Verification items for the finished model (mm, model axes). A direction names the side the tool comes from. Coordinates: 2 decimals unless noted, no trailing zeros. Loops run counter-clockwise (first coordinate to the right, second up) from the corner with the lowest first, then second, coordinate; pieces in that order, holes last. Notation, with made-up numbers: (10.5, 83.5) - (32.5, 83.5) arc R22 ccw to (32.5, 110.5) - close; hole circle Ø3 at (36, 48). An arc over 180 degrees is marked (long way). Answer as CSV lines item,"result". Start each with the question number.
1. Material ranges on line 1 (Z direction, x = 12.7, y = 1.75); line 2 (Y direction, x = 7.5, z = 548) (3 decimals); line 3 (X direction, y = 23.8, z = 698.5), recorded low to high. Write a range as [from, to].
2. Release check for a two-part mould opening along X. For faces 3 (the flat face through (13, 3.175, 361)), 4 (the flat face through (24, 13, 711.2)), 5 (the flat face through (25.4, 13, 351)) record: pulls with the +X half, pulls with the -X half, needs draft (parallel to the pull), parting line crosses it, or undercut.
3. Gauge pin test, flat end, axial feed: P1, Ø4, axis at x = 12.7, z = 476.25, coming from the -Y side. Record the tip position at first contact, or that the pin passes through.
4. Cross-section at A-A (z = 141.5). Enter the section's corners in (x, y) (3 decimals).
5. Cross-section at B-B (y = 8.75). Enter the section's corners in (x, z) (3 decimals).
6. Set-up check for faces 1 (the flat face through (0, 13, 351)), 2 (the flat face through (22.225, 13, 361)): record each of +Z, -Z, +X, -X, +Y, -Y from which the full face is reachable in a straight line by a thin tool's end or side.
Autodesk Inventor part; units mm, degrees
ref_plane "YZ Plane" through (0, 0, 0) normal (1, 0, 0) x (0, 1, 0)
ref_plane "XZ Plane" through (0, 0, 0) normal (0, 1, 0) x (-1, 0, 0)
ref_plane "XY Plane" through (0, 0, 0) normal (0, 0, 1) x (1, 0, 0)
sketch "Sketch1" plane through (0, 0, 0) normal (0, 0, 1) x (1, 0, 0)
  line L0 (0, 0) -> (25.4, 0)
  line L1 (25.4, 0) -> (25.4, 25.4)
  line L2 (25.4, 25.4) -> (0, 25.4)
  line L3 (0, 25.4) -> (0, 0)
  dimension "d0" = 25.4
  dimension "d1" = 25.4
extrude "Extrusion1" add sketch "Sketch1" along normal blind 711.2
sketch "Sketch2" plane through (0, 25.4, 0) normal (0, 1, 0) x (1, 0, 0)
  line L0 (0, -711.2) -> (25.4, -711.2) construction
  line L1 (12.7, -711.2) -> (12.7, -698.5) construction
  circle A0 centre (12.7, -698.5) radius 2.5797
  line L2 (12.7, -711.2) -> (12.7, -476.25) construction
  circle A1 centre (12.7, -476.25) radius 2.5797
  line L3 (0, 0) -> (0, -711.2) construction
  line L4 (0, -355.6) -> (25.4, -355.6) construction
  circle A2 centre (12.7, -12.7) radius 2.5797
  circle A3 centre (12.7, -234.95) radius 2.5797
  dimension "d4" = 12.7
  dimension "d5" = 5.1594
  dimension "d6" = 234.95
  dimension "d7" = 5.1594
extrude "Extrusion2" cut sketch "Sketch2" against normal blind 711.2
sketch "Sketch3" plane through (0, 0, 711.2) normal (0, 0, 1) x (1, 0, 0)
  line L0 (25.4, 25.4) -> (0, 25.4)
  line L1 (25.4, 0) -> (25.4, 25.4)
  line L2 (0, 25.4) -> (0, 0)
  line L3 (0, 0) -> (25.4, 0)
  line L4 (3.175, 22.225) -> (22.225, 22.225)
  line L5 (22.225, 22.225) -> (22.225, 3.175)
  line L6 (22.225, 3.175) -> (3.175, 3.175)
  line L7 (3.175, 3.175) -> (3.175, 22.225)
  dimension "d10" = 3.175
extrude "Extrusion3" cut sketch "Sketch3" against normal blind 762 contours L4 L5 L6 L7
properties part number "bumper runner"
Values follow:
1,line 1,"z = [0, 10.12], [15.28, 232.37], [237.53, 473.67], [478.83, 695.92], [701.08, 711.2]"
1,line 2,"y = [0, 3.175], [22.225, 25.4]"
1,line 3,"x = [0, 10.12], [15.28, 25.4]"
2,face 3,"undercut"
2,face 4,"needs draft"
2,face 5,"pulls with the +X half"
3,P1,"passes through"
4,outline,"(0, 0) - (25.4, 0) - (25.4, 25.4) - (0, 25.4) - close; hole (3.175, 3.175) - (22.225, 3.175) - (22.225, 22.225) - (3.175, 22.225) - close"
5,outline,"(0, 0) - (3.175, 0) - (3.175, 711.2) - (0, 711.2) - close; (22.225, 0) - (25.4, 0) - (25.4, 711.2) - (22.225, 711.2) - close"
6,face 1,"+Z, -Z, -X, +Y, -Y"
6,face 2,"+Z, -Z"
